Autodesk Inventor part; units mm, degrees
ref_plane "YZ Plane" through (0, 0, 0) normal (1, 0, 0) x (0, 1, 0)
ref_plane "XZ Plane" through (0, 0, 0) normal (0, 1, 0) x (-1, 0, 0)
ref_plane "XY Plane" through (0, 0, 0) normal (0, 0, 1) x (1, 0, 0)
sketch "Sketch1" plane through (0, 0, 0) normal (0, 0, 1) x (1, 0, 0)
  circle A0 centre (0, 0) radius 8 construction
  circle A1 centre (0, 0) radius 16 construction
  line L0 (20, -8.2843) -> (8.2843, -20)
  line L1 (8.2843, -20) -> (-8.2843, -20)
  line L2 (-8.2843, -20) -> (-20, -8.2843)
  line L3 (-20, 8.2843) -> (-8.2843, 20)
  line L4 (-8.2843, 20) -> (8.2843, 20)
  line L5 (8.2843, 20) -> (20, 8.2843)
  line L6 (20, 8.2843) -> (20, -8.2843)
  line L7 (-7.7279, 5) -> (-20, 5)
  line L8 (-7.7279, -5) -> (-20, -5)
  circle A2 centre (0, 0) radius 4.2
  line L9 (-20, -8.2843) -> (-20, -5)
  line L10 (-20, 5) -> (-20, 8.2843)
  line L11 (28, -11.598) -> (11.598, -28)
  line L12 (11.598, -28) -> (-11.598, -28)
  line L13 (-11.598, -28) -> (-28, -11.598)
  line L14 (-28, -11.598) -> (-28, 11.598)
  line L15 (-28, 11.598) -> (-11.598, 28)
  line L16 (-11.598, 28) -> (11.598, 28)
  line L17 (11.598, 28) -> (28, 11.598)
  line L18 (28, 11.598) -> (28, -11.598)
  line L19 (9, -3.7279) -> (3.7279, -9)
  line L20 (3.7279, -9) -> (-3.7279, -9)
  line L21 (-3.7279, 9) -> (3.7279, 9)
  line L22 (3.7279, 9) -> (9, 3.7279)
  line L23 (9, 3.7279) -> (9, -3.7279)
  line L24 (-20, 5) -> (-20, -5) construction
  line L25 (-3.7279, 9) -> (-7.7279, 5)
  line L26 (-3.7279, -9) -> (-7.7279, -5)
  point P0 (-20, 0)
  dimension "d1" = 16
  dimension "d2" = 32
  dimension "d5" = 8.4
  dimension "d6" = 40
  dimension "d7" = 8
  dimension "d8" = 10
  dimension "d10" = 18
extrude "Extrusion1" add sketch "Sketch1" along normal blind 6
sketch "Sketch2" plane through (0, 0, 6) normal (0, 0, 1) x (1, 0, 0)
  circle A0 centre (0, 0) radius 4.2
  line L0 (11.598, 28) -> (-11.598, 28)
  line L1 (-11.598, 28) -> (-28, 11.598)
  line L2 (-28, 11.598) -> (-28, -11.598)
  line L3 (-28, -11.598) -> (-11.598, -28)
  line L4 (-11.598, -28) -> (11.598, -28)
  line L5 (-24.7487, 14.8492) -> (-28, 18.1005)
  line L6 (-28, 18.1005) -> (-28, 23.8995)
  line L7 (-28, 23.8995) -> (-23.8995, 28)
  line L8 (-23.8995, 28) -> (-18.1005, 28)
  line L9 (-18.1005, 28) -> (-14.8492, 24.7487)
  line L10 (-28, 21) -> (-21, 21) construction
  line L11 (-21, 28) -> (-21, 21) construction
  circle A1 centre (-21, 21) radius 3.2
  line L12 (-24.7487, 14.8492) -> (-14.8492, 24.7487)
  line L13 (-14.8492, -24.7487) -> (-18.1005, -28)
  line L14 (-18.1005, -28) -> (-23.8995, -28)
  line L15 (-23.8995, -28) -> (-28, -23.8995)
  line L16 (-28, -23.8995) -> (-28, -18.1005)
  line L17 (-28, -18.1005) -> (-24.7487, -14.8492)
  circle A2 centre (-21, -21) radius 3.2
  line L18 (-14.8492, -24.7487) -> (-24.7487, -14.8492)
  line L19 (24.7487, -14.8492) -> (28, -18.1005)
  line L20 (28, -18.1005) -> (28, -23.8995)
  line L21 (28, -23.8995) -> (23.8995, -28)
  line L22 (23.8995, -28) -> (18.1005, -28)
  line L23 (18.1005, -28) -> (14.8492, -24.7487)
  circle A3 centre (21, -21) radius 3.2
  line L24 (24.7487, -14.8492) -> (14.8492, -24.7487)
  line L25 (14.8492, 24.7487) -> (18.1005, 28)
  line L26 (18.1005, 28) -> (23.8995, 28)
  line L27 (23.8995, 28) -> (28, 23.8995)
  line L28 (28, 23.8995) -> (28, 18.1005)
  line L29 (28, 18.1005) -> (24.7487, 14.8492)
  circle A4 centre (21, 21) radius 3.2
  line L30 (14.8492, 24.7487) -> (24.7487, 14.8492)
  circle A5 centre (-21, 21) radius 6 construction
  point P0 (-19.799, 19.799)
  point P1 (-21, -28)
  point P2 (-28, -21)
  point P3 (28, -21)
  point P4 (21, -28)
  point P5 (21, 28)
  point P6 (28, 21)
  dimension "d13" = 14
  dimension "d14" = 7
  dimension "d15" = 6.4
  dimension "d18" = 360
  dimension "d22" = 12
extrude "Extrusion2" add sketch "Sketch2" against normal blind 6 contours L3 A2 L13 L14 L15 L16 L17 | L5 L6 L7 L8 L9 L1 A1 | L19 L20 L21 L22 L23 L24 A3 | L25 L26 L27 L28 L29 L30 A4
sketch "Sketch3" plane through (0, 0, 6) normal (0, 0, 1) x (1, 0, 0)
  line L0 (-17.8813, 21.7167) -> (-21.7167, 17.8813)
  arc A0 (-17.8813, 21.7167) -> (-21.7167, 17.8813) centre (-21, 21) ccw
  line L1 (-21.7167, -17.8813) -> (-17.8813, -21.7167)
  arc A1 (-21.7167, -17.8813) -> (-17.8813, -21.7167) centre (-21, -21) ccw
  arc A2 (17.8813, -21.7167) -> (21.7167, -17.8813) centre (21, -21) ccw
  line L2 (17.8813, -21.7167) -> (21.7167, -17.8813)
  arc A3 (21.7167, 17.8813) -> (17.8813, 21.7167) centre (21, 21) ccw
  line L3 (21.7167, 17.8813) -> (17.8813, 21.7167)
  circle A4 centre (-21, -21) radius 3.2
  circle A5 centre (-21, 21) radius 3.2
  circle A6 centre (21, 21) radius 3.2
  circle A7 centre (21, -21) radius 3.2
extrude "Extrusion3" cut sketch "Sketch3" against normal through all contours A5 L0 | A4 L1 | A7 L2 | A6 L3
properties part number "x_iddler_belt_bearing_mount"
Could you check a few things on this model? Use its own coordinates, in mm. A direction names the side the tool comes from. Round coordinates to 2 decimals unless told otherwise and drop trailing zeros. Loops run counter-clockwise (first coordinate to the right, second up) from the corner with the lowest first, then second, coordinate; pieces in that order, holes last. Notation, with made-up numbers: (71.25, 42) - (92.25, 42) arc R20 ccw to (92.25, 67) - close; hole circle Ø4 at (-18, 5). An arc over 180 degrees is marked (long way). Write item = value, one per line.
1) Imagine slicing it at A-A (x = -21). Please give me the cut outline in (y, z), and give its area (3 significant figures).
Computed:
outline = (-28, 0) - (-24.2, 0) - (-24.2, 6) - (-28, 6) - close; (-17.8, 0) - (17.8, 0) - (17.8, 6) - (-17.8, 6) - close; (24.2, 0) - (28, 0) - (28, 6) - (24.2, 6) - close
area = 259 mm2
2) Imagine slicing it at B-B (x = 0). Please give me the cut outline in (y, z).
Computed:
outline = (-28, 0) - (-20, 0) - (-20, 6) - (-28, 6) - close; (-9, 0) - (-4.2, 0) - (-4.2, 6) - (-9, 6) - close; (4.2, 0) - (9, 0) - (9, 6) - (4.2, 6) - close; (20, 0) - (28, 0) - (28, 6) - (20, 6) - close
3) Imagine slicing it at D-D (z = 4.8). Give the number of separate pieces and of enclosed holes in the cut face, and give its area (3 significant figures).
Computed:
separate_pieces = 1
enclosed_holes = 6
area = 1,890 mm2
4) On a 3-axis mill with a long thin cutter (end or side, diameter ignored), from which of +Z, -Z, +X, -X, +Y, -Y can I reach the whole of each face in a straight line? I mean faces 1 (the flat face through (26.4, -16.5, 3)), 2 (the flat face through (16.5, 26.4, 3)), 3 (the flat face through (-5.7, -7.03, 2.96)). Say none if no direction works.
Computed:
face_1 = +Z, -Z, +X
face_2 = +Z, -Z, +Y
face_3 = +Z, -Z
5) I'm going to push flat-ended pins straight in: P1, Ø1, axis at y = 17, z = 5, coming from the +X side; P2, Ø4, axis at x = 21, y = 21, coming from the -Z side; P3, Ø3, axis at x = -16.5, z = 4.5, coming from the +Y side; P4, Ø3, axis at x = -13.5, z = 4, coming from the -Y side. Where does each tip first touch, or does it pass through?
Computed:
P1 = 27.4
P2 = through
P3 = 27.9
P4 = -27.6
6) If we mould it in two halves opening along Y, with no side actions, what happens to faces 4 (the flat face through (6.4, -6.33, 2.96)), 5 (the flat face through (26, -25.9, 3)), 6 (the flat face through (25.9, 26, 3))? For each: pulls with the +Y half, pulls with the -Y half, needs draft (parallel to the pull), parting line crosses it, or undercut.
Computed:
face_4 = undercut
face_5 = pulls with the -Y half
face_6 = pulls with the +Y half
7) I need wall thicknesses on line 1 along Y through (x, z) = (21, 3.2); line 2 along Y through (x, z) = (0, 3.25). Which ranges of each line are inside material? Lowest first, please. Write a range as from..to.
Computed:
line_1 = -28..-24.2, -17.8..17.8, 24.2..28
line_2 = -28..-20, -9..-4.2, 4.2..9, 20..28
